```python
from build123d import *

# Parameters (mm, degrees)
F0_W           = 126.7115995288
F0_H           = 131.4364373684
F1_DEPTH       = 5
F3_D           = 8.8
F3_CBORE_D     = 14.25
F3_CBORE_DEPTH = 3
F2_R           = 35
F4_DEPTH       = 50
F5_W           = 92.5968140364
F5_H           = 95.7502674907
F5_R           = 40
F5_R_2         = 35
F7_DEPTH       = 5
F9_DEPTH       = 18
F10_DEPTH      = 25
F11_D          = 8.8
F11_DEPTH      = 20
F11_TIP        = 2.6437867237
F12_R          = 3
F13_R          = 5


with BuildPart() as f1:
    # F0 (on Top) → F1 (new body)
    with BuildSketch(Plane.XY):
        with Locations((0.4295296967, -8.5906162858)):
            Rectangle(F0_W, F0_H)
    extrude(amount=F1_DEPTH)

    # F3 (through all)
    with Locations(Plane.XY.offset(5)):
        with Locations((-38.8249626095, 32.1276023984), (39.6840220029, 32.1276023984), (39.6840220029, -49.30883497), (-38.8249626095, -49.30883497)):
            CounterBoreHole(F3_D / 2, F3_CBORE_D / 2, F3_CBORE_DEPTH)

    # F2 (on face) → F4 (join)
    with BuildSketch(Plane.XY.offset(5)):
        with BuildLine():
            ThreePointArc((27.7619395928, 19.7609679006), (0.3092398069, 30.9626422773), (-27.3133733823, 20.1867676043))
            ThreePointArc((-27.3133733823, 20.1867676043), (-39.9988046164, -8.7269225322), (-27.7619395928, -37.8332925789))
            ThreePointArc((-27.7619395928, -37.8332925789), (0.3092398069, -49.0349669555), (28.2038686691, -37.4006082547))
            ThreePointArc((28.2038686691, -37.4006082547), (36.9334181113, -24.3959353393), (40, -9.0361623391))
            ThreePointArc((40, -9.0361623391), (36.8135680403, 6.6086837178), (27.7619395928, 19.7609679006))
        make_face()
        with Locations((0, -9.0361623391)):
            Circle(F2_R, mode=Mode.SUBTRACT)
    extrude(amount=F4_DEPTH)

    # F5 (on face) → F7 (join)
    with BuildSketch(Plane.XY.offset(55)):
        with Locations((0, -9.0361623391)):
            Rectangle(F5_W, F5_H)
        with Locations((0, -9.0361623391)):
            Circle(F5_R, mode=Mode.SUBTRACT)
        with Locations((0, -9.0361623391)):
            Circle(F5_R)
        with Locations((0, -9.0361623391)):
            Circle(F5_R_2, mode=Mode.SUBTRACT)
        with Locations((0, -9.0361623391)):
            Circle(F5_R_2)
    extrude(amount=F7_DEPTH)

    # F8 (on face) → F9 (join)
    with BuildSketch(Plane.XY.offset(60)):
        with BuildLine():
            Line((39.9663936465, 11.7301873131), (27.9663936465, 11.7301873131))
            Line((27.9663936465, 11.7301873131), (22.0274506375, -27.6131587349))
            ThreePointArc((22.0274506375, -27.6131587349), (17.9883204303, -34.9185557428), (10.1618760514, -37.8220306709))
            Line((10.1618760514, -37.8220306709), (0, -37.8220306709))
            Line((0, -37.8220306709), (-8.5433648964, -37.8220306709))
            ThreePointArc((-8.5433648964, -37.8220306709), (-16.1873438252, -35.0724136975), (-20.328320386, -28.0836283605))
            Line((-20.328320386, -28.0836283605), (-27.9462388724, 11.6125699067))
            Line((-27.9462388724, 11.6125699067), (-39.9462388724, 11.6125699067))
            Line((-39.9462388724, 11.6125699067), (-39.9462388724, -44.3874300933))
            Line((-39.9462388724, -44.3874300933), (39.9663936465, -44.2698126869))
            Line((39.9663936465, -44.2698126869), (39.9663936465, 11.7301873131))
        make_face()
    extrude(amount=F9_DEPTH)

    # F8 (on face) → F10 (join)
    with BuildSketch(Plane.XY.offset(60)):
        with BuildLine():
            Line((39.9663936465, 11.7301873131), (27.9663936465, 11.7301873131))
            Line((27.9663936465, 11.7301873131), (22.0274506375, -27.6131587349))
            ThreePointArc((22.0274506375, -27.6131587349), (17.9883204303, -34.9185557428), (10.1618760514, -37.8220306709))
            Line((10.1618760514, -37.8220306709), (0, -37.8220306709))
            Line((0, -37.8220306709), (-8.5433648964, -37.8220306709))
            ThreePointArc((-8.5433648964, -37.8220306709), (-16.1873438252, -35.0724136975), (-20.328320386, -28.0836283605))
            Line((-20.328320386, -28.0836283605), (-27.9462388724, 11.6125699067))
            Line((-27.9462388724, 11.6125699067), (-39.9462388724, 11.6125699067))
            Line((-39.9462388724, 11.6125699067), (-39.9462388724, -44.3874300933))
            Line((-39.9462388724, -44.3874300933), (39.9663936465, -44.2698126869))
            Line((39.9663936465, -44.2698126869), (39.9663936465, 11.7301873131))
        make_face()
    extrude(amount=F10_DEPTH)

    # F11
    with Locations(Plane.XY.offset(60)):
        with Locations((-34.6936167909, 26.8389714062), (34.6936167909, 26.8389714062)):
            Hole(F11_D / 2, depth=F11_DEPTH)
            with Locations((0, 0, -(F11_DEPTH + F11_TIP / 2))):  # 118° drill point
                Cone(0, F11_D / 2, F11_TIP, mode=Mode.SUBTRACT)

    # F12
    f12_edges = [f1.edges().sort_by_distance(p)[0] for p in [
        (27.76194, 19.760968, 5),
        (0.010077, -44.328621, 60),
        (39.966394, -16.269813, 60),
        (33.966394, 11.730187, 60),
        (-33.946239, 11.61257, 60),
        (-39.946239, -16.38743, 60),
        (-24.13728, -8.235529, 60),
        (17.98832, -34.918556, 85),
        (39.966394, -16.269813, 85),
        (0.010077, -44.328621, 85),
        (-39.946239, -16.38743, 85),
        (-33.946239, 11.61257, 85),
        (33.966394, 11.730187, 85),
        (27.76194, 19.760968, 55),
    ]]
    fillet(f12_edges, radius=F12_R)

    # F13
    f13_edges = [f1.edges().sort_by_distance(p)[0] for p in [
        (63.785329, 57.127602, 2.5),
        (-62.92627, 57.127602, 2.5),
        (63.785329, -74.308835, 2.5),
        (46.298407, -56.911296, 57.5),
        (46.298407, 38.838971, 57.5),
        (-46.298407, 38.838971, 57.5),
        (-62.92627, -74.308835, 2.5),
        (-46.298407, -56.911296, 57.5),
    ]]
    fillet(f13_edges, radius=F13_R)


solid = f1.part
```
Design review of the part built by this model. Coordinates are the model's own, in mm. A direction names the side the tool comes from. Round coordinates to 2 decimals unless told otherwise and drop trailing zeros. Order: outer loops, then holes, each group sorted by start corner. A loop starts at its lowest first (then second) coordinate and runs counter-clockwise, first axis right, second up. Notation, with made-up numbers: M 58.5,35 L 90.5,35 A21 ccw 90.5,55 Z; hole C 55,28.5 d9. An arc over 180 degrees is marked long. Put each result on its own line as item: value.
Q1. Draft analysis for pull direction Z (two halves, no side actions). For faces 6 (the face through (-23.542, -6.553, 60.855)), 7 (the face through (-44.87, -55.41, 57.54)), 8 (the face through (0, 36, 5)), state which applies: released by +Z, released by -Z, zero draft, split by the parting line, or undercut.
Reported:
face 6: released by +Z
face 7: zero draft
face 8: undercut
Q2. Insertion check: pin 1 Ø16.5 at (x, y) = (-38.82, 32.13) entering from +Z; pin 2 Ø4 at (x, z) = (-17.5, 12.5) entering from -Y; pin 3 Ø13 at (x, y) = (-38.82, -49.31) entering from +Z. Each pin has a flat end and moves straight along its axis. Give the tip position at first contact, or say it passes through.
Reported:
pin 1: z = 60
pin 2: y = -45.91
pin 3: z = 84.63
Q3. Consider section A-A (z = 27.5). State the section outline as (x, y) points, and give its area (3 significant figures).
Reported:
outline: C 0,-9.04 d80; hole C 0,-9.04 d70
area: 1,180 mm²
Q4. Machinability: for faces 1 (the face through (-24.084, -8.513, 72.367)), 2 (the face through (-1, -56.911, 57)), 3 (the face through (44.795, 37.413, 57.535)), 4 (the face through (-40.37, -56.264, 3.521)), 5 (the face through (39.966, -17, 72)), which of the approach directions +Z, -Z, +X, -X, +Y, -Y give a long, thin tool a straight path to every point of the face, cutting with its end or side? Answer none if there is none.
Reported:
face 1: +Z, +Y
face 2: +Z, +X, -X, -Y
face 3: +Z, +X, +Y
face 4: none
face 5: +Z, +X, +Y, -Y
Q5. Consider section B-B (y = 43.5). State the section outline as (x, z) points.
Reported:
outline: M -62.93,0 L 63.79,0 L 63.79,5 L -62.93,5 Z
Q6. To check wall thickness, follow line 1 (Z direction, x = -19, y = 9.5); line 2 (Y direction, x = -30, z = 81.5); line 3 (Z direction, x = 54, y = -0.5). State the ranges of each line that lie inside material, in increasing order.
Reported:
line 1: 0 to 5, 55 to 60
line 2: -44.37 to 11.61
line 3: 0 to 5
